```python
from build123d import *

# Parameters (mm, degrees)
F1_DEPTH = 5


with BuildPart() as f1:
    # F0 (on Top) → F1 (new body)
    with BuildSketch(Plane.XY):
        with BuildLine():
            ThreePointArc((-10.1051355834, 0), (-9.2996792316, 1.9445436483), (-7.3551355834, 2.75))
            Line((-7.3551355834, 2.75), (-4.8056258266, 2.75))
            ThreePointArc((-4.8056258266, 2.75), (-5.9858291896, 3.4910600109), (-7.3551355834, 3.75))
            ThreePointArc((-7.3551355834, 3.75), (-11.1051355834, 0), (-7.3551355834, -3.75))
            ThreePointArc((-7.3551355834, -3.75), (-5.9858291896, -3.4910600109), (-4.8056258266, -2.75))
            Line((-4.8056258266, -2.75), (-7.3551355834, -2.75))
            ThreePointArc((-7.3551355834, -2.75), (-9.2996792316, -1.9445436483), (-10.1051355834, 0))
        make_face()
        with BuildLine():
            ThreePointArc((-7.3551355834, 3.75), (-5.9858291896, 3.4910600109), (-4.8056258266, 2.75))
            Line((-4.8056258266, 2.75), (2.8953546598, 2.75))
            ThreePointArc((2.8953546598, 2.75), (4.0755580229, 3.4910600109), (5.4448644166, 3.75))
            Line((5.4448644166, 3.75), (-7.3551355834, 3.75))
        make_face()
        with BuildLine():
            ThreePointArc((5.4448644166, 3.75), (4.0755580229, 3.4910600109), (2.8953546598, 2.75))
            Line((2.8953546598, 2.75), (5.4448644166, 2.75))
            ThreePointArc((5.4448644166, 2.75), (7.3894080649, 1.9445436483), (8.1948644166, 0))
            ThreePointArc((8.1948644166, 0), (7.3894080649, -1.9445436483), (5.4448644166, -2.75))
            Line((5.4448644166, -2.75), (2.8953546598, -2.75))
            ThreePointArc((2.8953546598, -2.75), (4.0755580229, -3.4910600109), (5.4448644166, -3.75))
            ThreePointArc((5.4448644166, -3.75), (8.0965148461, -2.6516504294), (9.1948644166, 0))
            ThreePointArc((9.1948644166, 0), (8.0965148461, 2.6516504294), (5.4448644166, 3.75))
        make_face()
        with BuildLine():
            Line((2.8953546598, -2.75), (-4.8056258266, -2.75))
            ThreePointArc((-4.8056258266, -2.75), (-5.9858291896, -3.4910600109), (-7.3551355834, -3.75))
            Line((-7.3551355834, -3.75), (5.4448644166, -3.75))
            ThreePointArc((5.4448644166, -3.75), (4.0755580229, -3.4910600109), (2.8953546598, -2.75))
        make_face()
    extrude(amount=F1_DEPTH)


solid = f1.part
```
Geometry check sheet. Reference: the model listing, model coordinates, mm. A direction names the side the tool comes from. Round coordinates to 2 decimals unless told otherwise and drop trailing zeros. Loops run counter-clockwise (first coordinate to the right, second up) from the corner with the lowest first, then second, coordinate; pieces in that order, holes last. Notation, with made-up numbers: M -14.75,24 L 18.25,24 A24 cw 18.25,40 Z; hole C 86.25,68 d11. An arc over 180 degrees is marked long. Return JSON: item names as keys, results as strings. Group by question number.
(1) Set-up check for faces 1 (the face through (9.194, -0.082, 2.465)), 2 (the face through (-1, -2.75, 2)): record each of +Z, -Z, +X, -X, +Y, -Y from which the full face is reachable in a straight line by a thin tool's end or side.
(2) Section check C-C, the plane y = 2.5. Enter the section's corners in (x, z).
(3) Section check A-A, the plane x = -3.5. Enter the section's corners in (y, z), and give its area (3 significant figures).
(4) Mould release check, pull along X, two halves, no side actions. Record for faces 3 (the face through (-1, -3.75, 2)), 4 (the face through (-11.104, 0.082, 2.465)), 5 (the face through (-1, 2.75, 2)): pulls with the +X half, pulls with the -X half, needs draft (parallel to the pull), parting line crosses it, or undercut.
(5) Section check B-B, the plane z = 3.9. Enter the section's corners in (x, y), and give its area (3 significant figures).
(6) Scan lines: line 1 along Y through (x, z) = (-1.25, 4.75); line 2 along X through (y, z) = (-0.75, 1.2); line 3 along X through (y, z) = (1.75, 1.65). Record each from-to range of solid material in increasing order. Write a range as [from, to].
(7) Go/stop test with a flat-tipped pin: pin 1 (3 mm diameter, centred on x = 5.5, y = -1, fed in from -Z). Record where the tip stops, or that it passes through.
Data:
{
 "1": {"face 1": "+Z, -Z, +X", "face 2": "+Z, -Z"},
 "2": {"outline": "M -10.15,0 L -8.5,0 L -8.5,5 L -10.15,5 Z; M 6.59,0 L 8.24,0 L 8.24,5 L 6.59,5 Z"},
 "3": {"outline": "M -3.75,0 L -2.75,0 L -2.75,5 L -3.75,5 Z; M 2.75,0 L 3.75,0 L 3.75,5 L 2.75,5 Z", "area": "10.0 mm²"},
 "4": {"face 3": "needs draft", "face 4": "pulls with the -X half", "face 5": "undercut"},
 "5": {"outline": "M -7.36,-3.75 L 5.44,-3.75 A3.75 ccw 5.44,3.75 L -7.36,3.75 A3.75 ccw Z; hole M -7.36,-2.75 L 5.44,-2.75 A2.75 ccw 5.44,2.75 L -7.36,2.75 A2.75 ccw Z", "area": "46.0 mm²"},
 "6": {"line 1": "[-3.75, -2.75], [2.75, 3.75]", "line 2": "[-11.03, -10], [8.09, 9.12]", "line 3": "[-10.67, -9.48], [7.57, 8.76]"},
 "7": {"pin 1": "through"}
}
